from build123d import *

# Parameters (mm, degrees)
SKETCH1_R           = 12.5
SKETCH1_R_2         = 1.5
BOSS_EXTRUDE1_DEPTH = 1
SKETCH3_R           = 13.5
SKETCH3_R_2         = 12.5
BOSS_EXTRUDE2_DEPTH = 1
BOSS_EXTRUDE3_DEPTH = 2


with BuildPart() as part:
    # Sketch1 → Boss-Extrude1 (new body)
    with BuildSketch(Plane(origin=(0, 0, 0), x_dir=(1, 0, 0), z_dir=(0, 1, 0))):
        with BuildLine():
            Line((-12, -14), (12, -14))
            ThreePointArc((12, -14), (13.414213562, -13.414213562), (14, -12))
            Line((14, -12), (14, 12))
            ThreePointArc((14, 12), (13.414213562, 13.414213562), (12, 14))
            Line((12, 14), (-12, 14))
            ThreePointArc((-12, 14), (-13.414213562, 13.414213562), (-14, 12))
            Line((-14, 12), (-14, -12))
            ThreePointArc((-14, -12), (-13.414213562, -13.414213562), (-12, -14))
        make_face()
        Circle(SKETCH1_R, mode=Mode.SUBTRACT)
        with Locations((-12, 12)):
            Circle(SKETCH1_R_2, mode=Mode.SUBTRACT)
        with Locations((12, 12)):
            Circle(SKETCH1_R_2, mode=Mode.SUBTRACT)
        with Locations((12, -12)):
            Circle(SKETCH1_R_2, mode=Mode.SUBTRACT)
        with Locations((-12, -12)):
            Circle(SKETCH1_R_2, mode=Mode.SUBTRACT)
    extrude(amount=BOSS_EXTRUDE1_DEPTH)

    # Sketch3 → Boss-Extrude2 (add)
    with BuildSketch(Plane(origin=(0, 1, 0), x_dir=(1, 0, 0), z_dir=(0, 1, 0))):
        Circle(SKETCH3_R)
        Circle(SKETCH3_R_2, mode=Mode.SUBTRACT)
    extrude(amount=BOSS_EXTRUDE2_DEPTH)

    # Sketch4 → Boss-Extrude3 (add)
    with BuildSketch(Plane(origin=(0, 0, 0), x_dir=(1, 0, 0), z_dir=(0, 1, 0))):
        with BuildLine():
            Line((-4.454043904, 1.306562965), (0.181881395, 12.498676696))
            ThreePointArc((0.181881395, 12.498676696), (0.711234958, 12.47974939), (1.239311378, 12.438412572))
            Line((1.239311378, 12.438412572), (-2.225605116, 4.073364181))
            Line((-2.225605116, 4.073364181), (8.966508616, 8.70928948))
            ThreePointArc((8.966508616, 8.70928948), (9.327434483, 8.321596359), (9.671611356, 7.918960398))
            Line((9.671611356, 7.918960398), (1.306562965, 4.454043904))
            Line((1.306562965, 4.454043904), (12.498676696, -0.181881395))
            ThreePointArc((12.498676696, -0.181881395), (12.47974939, -0.711234958), (12.438412572, -1.239311378))
            Line((12.438412572, -1.239311378), (4.073364181, 2.225605116))
            Line((4.073364181, 2.225605116), (8.70928948, -8.966508616))
            ThreePointArc((8.70928948, -8.966508616), (8.321596359, -9.327434483), (7.918960398, -9.671611356))
            Line((7.918960398, -9.671611356), (4.454043904, -1.306562965))
            Line((4.454043904, -1.306562965), (-0.181881395, -12.498676696))
            ThreePointArc((-0.181881395, -12.498676696), (-0.711234958, -12.47974939), (-1.239311378, -12.438412572))
            Line((-1.239311378, -12.438412572), (2.225605116, -4.073364181))
            Line((2.225605116, -4.073364181), (-8.966508616, -8.70928948))
            ThreePointArc((-8.966508616, -8.70928948), (-9.327434483, -8.321596359), (-9.671611356, -7.918960398))
            Line((-9.671611356, -7.918960398), (-1.306562965, -4.454043904))
            Line((-1.306562965, -4.454043904), (-12.498676696, 0.181881395))
            ThreePointArc((-12.498676696, 0.181881395), (-12.47974939, 0.711234958), (-12.438412572, 1.239311378))
            Line((-12.438412572, 1.239311378), (-4.073364181, -2.225605116))
            Line((-4.073364181, -2.225605116), (-8.70928948, 8.966508616))
            ThreePointArc((-8.70928948, 8.966508616), (-8.321596359, 9.327434483), (-7.918960398, 9.671611356))
            Line((-7.918960398, 9.671611356), (-4.454043904, 1.306562965))
        make_face()
    extrude(amount=BOSS_EXTRUDE3_DEPTH)


solid = part.part
Geometry check sheet. Reference: the model listing, model coordinates, mm. A direction names the side the tool comes from. Give positions to 0.01 mm unless a question says otherwise; leave off trailing zeros. Order: outer loops, then holes, each group sorted by start corner. A loop starts at its lowest first (then second) coordinate and runs counter-clockwise, first axis right, second up. Notation, with made-up numbers: (22, -1.5) - (36, -1.5) arc R25 cw to (36, 35.5) - close; hole circle Ø11 at (55, -9). An arc over 180 degrees is marked (long way). Answer as a JSON object with one key per item and string values.
(1) Tool access check on faces 4 (the flat face through (-8.31, 0.99, 0.47)), 5 (the flat face through (0, 0, 0)), 6 (the flat face through (-13, 1, 5)). Record the directions out of +Z, -Z, +X, -X, +Y, -Y that give a thin tool (end or side, any length) a straight path to the whole face; none if there is none.
Report:
{"face 4": "+Y, -Y", "face 5": "+Z, -Z, +X, -X, -Y", "face 6": "+Y"}
(2) Draft check along X on faces 1 (the flat face through (0.2, 0.5, -14)), 2 (the flat face through (-14, 0.5, -0.2)), 3 (the cylindrical face through (-13.5, 0.49, -12.07)). Enter one of: released by +X, released by -X, zero draft, split by the parting line, or undercut.
Report:
{"face 1": "zero draft", "face 2": "released by -X", "face 3": "undercut"}
(3) Cross-section at B-B (y = 1.7). State how many separate pieces and enclosed holes the cut face has, then the cut area to 3 significant figures.
Report:
{"separate pieces": "1", "enclosed holes": "8", "area": "227 mm^2"}
(4) Material ranges on line 1 (X direction, y = 1.6, z = -5.5); line 2 (X direction, y = 0.25, z = 9); line 3 (X direction, y = 0.5, z = -2), recorded low to high.
Report:
{"line 1": "-12.33 to -11.22, -7.27 to -6.19, -2.72 to -1.63, 1.22 to 3.83, 11.22 to 12.33", "line 2": "-14 to -8.67, 0.18 to 1.27, 7.64 to 14", "line 3": "-14 to -12.34, -5.82 to -4.74, -4.17 to 4.17, 4.62 to 7.23, 12.34 to 14"}
(5) Cross-section at D-D (z = 5.25). Record the cut outline in (x, y).
Report:
{"outline": "(-14, 0) - (-11.34, 0) - (-11.34, 2) - (-12.44, 2) - (-12.44, 1) - (-14, 1) - close; (-3.23, 0) - (-0.62, 0) - (-0.62, 2) - (-3.23, 2) - close; (1.74, 0) - (2.82, 0) - (2.82, 2) - (1.74, 2) - close; (6.09, 0) - (7.17, 0) - (7.17, 2) - (6.09, 2) - close; (11.34, 0) - (14, 0) - (14, 1) - (12.44, 1) - (12.44, 2) - (11.34, 2) - close"}
(6) Depth check by flat-ended pin: pin 1 Ø5 at (x, z) = (12, 12) entering from +Y. Enter the tip coordinate at first touch or a pass-through.
Report:
{"pin 1": "y = 1"}
(7) Cross-section at C-C (x = 3.75). Record the cut outline in (y, z), then the cut area to 3 significant figures.
Report:
{"outline": "(0, -14) - (1, -14) - (1, -12.97) - (2, -12.97) - (2, -11.92) - (0, -11.92) - close; (0, -6.55) - (2, -6.55) - (2, -5.47) - (0, -5.47) - close; (0, -3.44) - (2, -3.44) - (2, 3.01) - (0, 3.01) - close; (0, 11.92) - (2, 11.92) - (2, 12.97) - (1, 12.97) - (1, 14) - (0, 14) - close", "area": "21.3 mm^2"}
(8) Cross-section at A-A (z = 10). Record the cut outline in (x, y), then the cut area to 3 significant figures.
Report:
{"outline": "(-14, 0) - (-7.5, 0) - (-7.5, 2) - (-9.07, 2) - (-9.07, 1) - (-14, 1) - close; (-0.23, 0) - (0.85, 0) - (0.85, 2) - (-0.23, 2) - close; (7.5, 0) - (14, 0) - (14, 1) - (9.07, 1) - (9.07, 2) - (7.5, 2) - close", "area": "18.3 mm^2"}
